Design review of the part built by this model. Coordinates are the model's own, in mm. A direction names the side the tool comes from. Coordinates: 2 decimals unless noted, no trailing zeros. Write each loop counter-clockwise with the first axis right and the second up, starting at its lowest first coordinate (ties: lowest second). Pieces come first, ordered by that corner, then holes. Notation, with made-up numbers: (25, -36.5) -> (35, -36.5) arc R16 ccw to (35, -16.5) -> close; hole circle Ø8 at (6.5, 21.25). An arc over 180 degrees is marked (long way). Return JSON: item names as keys, results as strings. Group by question number.
from build123d import *

# Parameters (mm, degrees)
BOSS_EXTRUDE1_DEPTH = 4
SKETCH2_R           = 4
CUT_EXTRUDE2_DEPTH  = 5
SKETCH5_R           = 1.7
CUT_EXTRUDE3_DEPTH  = 5
FILLET1_R           = 5
FILLET2_R           = 5
FILLET3_R           = 1


with BuildPart() as part:
    # Sketch3 → Boss-Extrude1 (new body)
    with BuildSketch(Plane.XY):
        with BuildLine():
            Line((-7.5, -21.213203436), (-7.5, -45))
            Line((-7.5, -45), (-22.5, -45))
            Line((-22.5, -45), (-22.5, -26.809513237))
            ThreePointArc((-22.5, -26.809513237), (0, 35), (22.5, -26.809513237))
            Line((22.5, -26.809513237), (22.5, -45))
            Line((22.5, -45), (7.5, -45))
            Line((7.5, -45), (7.5, -21.213203436))
            ThreePointArc((7.5, -21.213203436), (17.734611105, -13.846789121), (22.398843942, -2.131147595))
            ThreePointArc((22.398843942, -2.131147595), (23.640685275, -2.41653339), (24.836154938, -2.857517782))
            ThreePointArc((24.836154938, -2.857517782), (0, 25), (-24.836154938, -2.857517782))
            ThreePointArc((-24.836154938, -2.857517782), (-23.640685275, -2.41653339), (-22.398843942, -2.131147595))
            ThreePointArc((-22.398843942, -2.131147595), (-17.734611105, -13.846789121), (-7.5, -21.213203436))
        make_face()
    extrude(amount=BOSS_EXTRUDE1_DEPTH)

    # Sketch2 → Cut-Extrude2 (cut, through all)
    with BuildSketch(Plane.XY):
        with Locations((0, 26.5)):
            Circle(SKETCH2_R)
        with Locations((-20.784609691, -12)):
            Circle(SKETCH2_R)
        with Locations((20.784609691, -12)):
            Circle(SKETCH2_R)
    extrude(amount=CUT_EXTRUDE2_DEPTH, mode=Mode.SUBTRACT)

    # Sketch5 → Cut-Extrude3 (cut, through all)
    with BuildSketch(Plane.XY):
        with Locations((-15, -37.5)):
            Circle(SKETCH5_R)
        with Locations((15, -37.5)):
            Circle(SKETCH5_R)
    extrude(amount=CUT_EXTRUDE3_DEPTH, mode=Mode.SUBTRACT)

    # Fillet1
    fillet1_edges = [part.edges().sort_by_distance(p)[0] for p in [
        (22.5, -45, 2),
        (-22.5, -45, 2),
    ]]
    fillet(fillet1_edges, radius=FILLET1_R)

    # Fillet2
    fillet2_edges = [part.edges().sort_by_distance(p)[0] for p in [
        (22.5, -26.809513237, 2),
        (7.5, -45, 2),
        (7.5, -21.213203436, 2),
        (-7.5, -21.213203436, 2),
        (-7.5, -45, 2),
        (-22.5, -26.809513237, 2),
    ]]
    fillet(fillet2_edges, radius=FILLET2_R)

    # Fillet3
    fillet3_edges = [part.edges().sort_by_distance(p)[0] for p in [
        (22.398843942, -2.131147595, 2),
        (24.836154938, -2.857517782, 2),
        (-24.836154938, -2.857517782, 2),
        (-22.398843942, -2.131147595, 2),
    ]]
    fillet(fillet3_edges, radius=FILLET3_R)


solid = part.part
Q1. We need section D-D on z = 1.2. State how many separate pieces and enclosed holes the cut face has, plus the area to 3 significant figures.
Q2. We need section C-C on x = -14.5. Write out the cut boundary in (y, z).
Q3. Wall thickness on L1, parallel to Y at x = -15, z = 2.7; L2, parallel to X at y = -37.5, z = 2.55; L3, parallel to X at y = 0.5, z = 0.75 (3 decimals): over which ranges is each line inside the solid? List them lowest first.
Q4. For P1, Ø1.2, axis at y = -35, z = 2.5, coming from the +X side; P2, Ø2, axis at x = -11, z = 2.5, coming from the +Y side; P3, Ø1, axis at x = 24.5, z = 0.5, coming from the +Y side, all flat-tipped, find the tip position at first contact; note any pin that passes through.
Q5. For faces 4 (the cylindrical face through (-21.79, -5.61, 1.97)), 5 (the flat face through (22.5, -34, 2)), 6 (the flat face through (15, -45, 2)), 7 (the flat face through (-22.5, -35, 2)), 8 (the cylindrical face through (-9, -43.57, 2.03)), list the 3-axis set-ups (+Z, -Z, +X, -X, +Y, -Y) from which the entire face can be reached by the end or side of a thin tool; tool diameter is ignored.
Q6. The part is to be moulded in two halves that separate along Y. For faces 1 (the flat face through (8.3, -22.2, 4)), 2 (the cylindrical face through (-24.304, -13.901, 1.972)), 3 (the cylindrical face through (9, -43.57, 2.03)), say which applies: +Y half, -Y half, draft (parallel to the pull), parting line (faces both ways), or undercut.
Q7. We need section A-A on y = -37.5. Write out the cut boundary in (x, z).
Q8. We need section B-B on y = 0. Write out the cut boundary in (x, z), plus the area to 3 significant figures.
Findings below:
{
 "1": {"separate pieces": "1", "enclosed holes": "2", "area": "2,130 mm^2"},
 "2": {"outline": "(-45, 0) -> (-39.12, 0) -> (-39.12, 4) -> (-45, 4) -> close; (-35.88, 0) -> (-17.2, 0) -> (-17.2, 4) -> (-35.88, 4) -> close; (20.37, 0) -> (31.86, 0) -> (31.86, 4) -> (20.37, 4) -> close"},
 "3": {"L1": "y = -45 to -39.2, -35.8 to -16.77, 20 to 31.62", "L2": "x = -22.5 to -16.7, -13.3 to -7.5, 7.5 to 13.3, 16.7 to 22.5", "L3": "x = -34.996 to -24.995, 24.995 to 34.996"},
 "4": {"P1": "stops at x = 22.5", "P2": "stops at y = 33.54", "P3": "stops at y = 25.48"},
 "5": {"face 4": "+Z, -Z", "face 5": "+Z, -Z, +X, -Y", "face 6": "+Z, -Z, +X, -X, -Y", "face 7": "+Z, -Z, -X, -Y", "face 8": "+Z, -Z, -Y"},
 "6": {"face 1": "draft", "face 2": "undercut", "face 3": "-Y half"},
 "7": {"outline": "(-22.5, 0) -> (-16.7, 0) -> (-16.7, 4) -> (-22.5, 4) -> close; (-13.3, 0) -> (-7.5, 0) -> (-7.5, 4) -> (-13.3, 4) -> close; (7.5, 0) -> (13.3, 0) -> (13.3, 4) -> (7.5, 4) -> close; (16.7, 0) -> (22.5, 0) -> (22.5, 4) -> (16.7, 4) -> close"},
 "8": {"outline": "(-35, 0) -> (-25, 0) -> (-25, 4) -> (-35, 4) -> close; (25, 0) -> (35, 0) -> (35, 4) -> (25, 4) -> close", "area": "80.0 mm^2"}
}
